Design review of the part shown in the three views and the two pictorial views. Dimensions are in mm from the part's minimum x, y and z. A direction names the side the tool comes from. Round coordinates to 2 decimals unless told otherwise and drop trailing zeros. Order: outer loops, then holes, each group sorted by start corner. A loop starts at its lowest first (then second) coordinate and runs counter-clockwise, first axis right, second up.
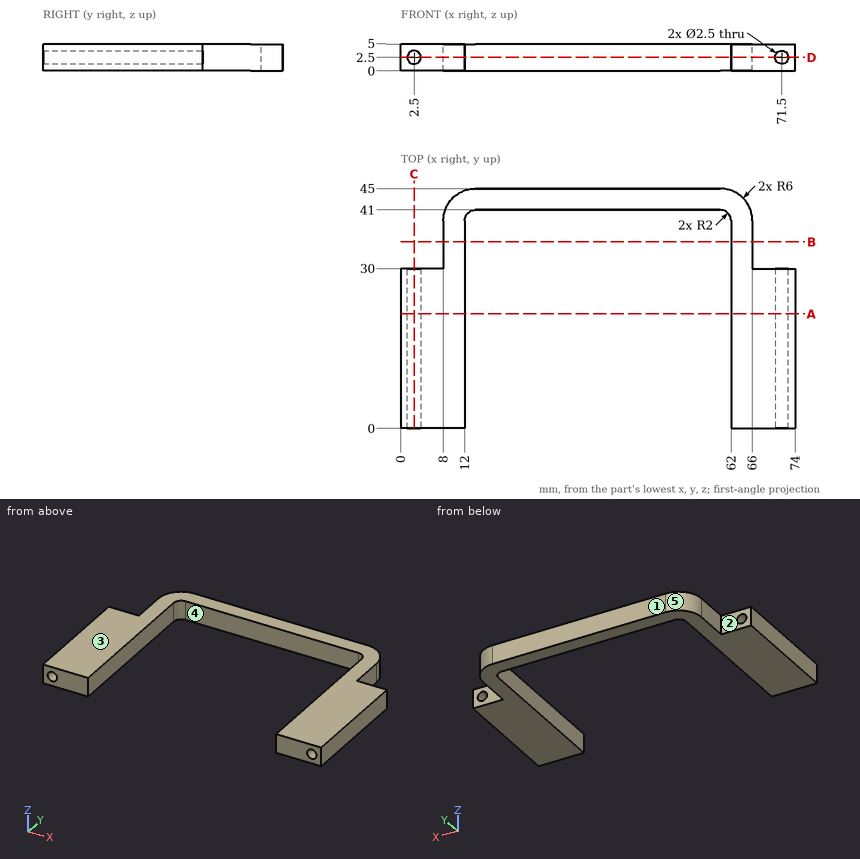
1) Take a section at D-D on z = 2.5. Give the boundary of the cut face in (x, y), plus the area to 3 significant figures.
Results:
outline: (0, 0) - (1.25, 0) - (1.25, 30) - (0, 30) - close; (3.75, 0) - (12, 0) - (12, 39) arc R2 cw to (14, 41) - (60, 41) arc R2 cw to (62, 39) - (62, 0) - (70.25, 0) - (70.25, 30) - (66, 30) - (66, 39) arc R6 ccw to (60, 45) - (14, 45) arc R6 ccw to (8, 39) - (8, 30) - (3.75, 30) - close; (72.75, 0) - (74, 0) - (74, 30) - (72.75, 30) - close
area: 876 mm2
2) Clearance check with flat-ended pins moving along their axes: P1, Ø2.5, axis at y = 33, z = 3.5, coming from the +X side; P2, Ø2, axis at y = 10.5, z = 3.5, coming from the -X side; P3, Ø2, axis at x = 71.5, z = 2.5, coming from the -Y side; P4, Ø2.5, axis at y = 36, z = 3.5, coming from the -X side. State where each tip first meets the part, or that it passes through.
Results:
P1: stops at x = 66
P2: stops at x = 0
P3: passes through
P4: stops at x = 8
3) Take a section at A-A on y = 21.5. Give the boundary of the cut face in (x, z).
Results:
outline: (0, 0) - (12, 0) - (12, 5) - (0, 5) - close; (62, 0) - (74, 0) - (74, 5) - (62, 5) - close; hole circle Ø2.5 at (2.5, 2.5); hole circle Ø2.5 at (71.5, 2.5)
4) To check wall thickness, follow line 1 along X through (y, z) = (8, 2.6); line 2 along X through (y, z) = (34.5, 2.95); line 3 along Z through (x, y) = (2.5, 14.75). State the ranges of each line that lie inside material, in increasing order.
Results:
line 1: x = 0 to 1.25, 3.75 to 12, 62 to 70.25, 72.75 to 74
line 2: x = 8 to 12, 62 to 66
line 3: z = 0 to 1.25, 3.75 to 5
5) The part is to be moulded in two halves that separate along X. For the marked faces 3, 4 and 5, say which applies: released by +X, released by -X, zero draft, split by the parting line, or undercut.
Results:
face 3: zero draft
face 4: undercut
face 5: released by -X
6) Take a section at C-C on x = 2.5. Give the boundary of the cut face in (y, z), plus the area to 3 significant figures.
Results:
outline: (0, 0) - (30, 0) - (30, 1.25) - (0, 1.25) - close; (0, 3.75) - (30, 3.75) - (30, 5) - (0, 5) - close
area: 75.0 mm2
7) For the marked faces 1 and 2, list the 3-axis set-ups (+Z, -Z, +X, -X, +Y, -Y) from which the entire face can be reached by the end or side of a thin tool; tool diameter is ignored.
Results:
face 1: +Z, -Z, +X, -X, +Y
face 2: +Z, -Z, -X, +Y
8) Take a section at B-B on y = 35. Give the boundary of the cut face in (x, z), plus the area to 3 significant figures.
Results:
outline: (8, 0) - (12, 0) - (12, 5) - (8, 5) - close; (62, 0) - (66, 0) - (66, 5) - (62, 5) - close
area: 40.0 mm2
